from build123d import *


with BuildPart() as part:
    # Эскиз1 → Повернуть1 (revolve)
    with BuildSketch(Plane.XY):
        with BuildLine():
            Line((13.062177826, 3.5), (32, 12.5))
            Line((32, 12.5), (42, 12.5))
            Line((42, 12.5), (60.937822174, 3.5))
            ThreePointArc((60.937822174, 3.5), (68.811733316, 6.761480784), (74, 0))
            Line((74, 0), (0, 0))
            ThreePointArc((0, 0), (5.188266684, 6.761480784), (13.062177826, 3.5))
        make_face()
    revolve(axis=Axis((0, 0, 0), (1, 0, 0)))

    # Эскиз4 → Вырез-Повернуть1 (revolve, cut)
    with BuildSketch(Plane(origin=(37, 0, 0), x_dir=(0, 0, -1), z_dir=(1, 0, 0))):
        Polygon((-7.5, 10), (7.5, 10), (7.5, 20), (15, 20), (15, 0), (-15, 0), (-15, 20), (-7.5, 20), align=None)
    revolve(axis=Axis((37, 0, 0), (0, 0, -1)), mode=Mode.SUBTRACT)


solid = part.part
Verification items for the finished model (mm, model axes). A direction names the side the tool comes from. Coordinates: 2 decimals unless noted, no trailing zeros. Order: outer loops, then holes, each group sorted by start corner. A loop starts at its lowest first (then second) coordinate and runs counter-clockwise, first axis right, second up.
Item 1: Depth check by flat-ended pin: pin 1 (3 mm diameter, centred on y = -2.5, z = -3.5, fed in from -X); pin 2 (1 mm diameter, centred on x = 8.5, z = 5.5, fed in from -Y); pin 3 (2 mm diameter, centred on x = 49.5, z = 3, fed in from -Y). Enter the tip coordinate at first touch or a pass-through.
Filled in:
pin 1: stops at x = 0.58
pin 2: stops at y = -4.69
pin 3: stops at y = -9.01
Item 2: Material ranges on L1, parallel to X at y = 0, z = 0.25; L2, parallel to Y at x = 31, z = 2.75; L3, parallel to X at y = 0, z = 3.25, recorded low to high.
Filled in:
L1: x = 0 to 27, 47 to 74
L2: y = -11.71 to -8, 8 to 11.71
L3: x = 0.8 to 27, 47 to 73.2
Item 3: Section check B-B, the plane y = 0. Enter the section's corners in (x, z).
Filled in:
outline: (13.06, -3.5) - (21.48, -7.5) - (27, -7.5) - (27, 7.5) - (21.48, 7.5) - (13.06, 3.5) arc R7 ccw (long way) to start; (47, -7.5) - (52.52, -7.5) - (60.94, -3.5) arc R7 ccw (long way) to (60.94, 3.5) - (52.52, 7.5) - (47, 7.5) - close
Item 4: Release check for a two-part mould opening along X. For faces 1 (the face through (26, 0, 7.5)), 2 (the face through (18.455, -4.811, -3.689)) record: +X half, -X half, draft (parallel to the pull), parting line (faces both ways), or undercut.
Filled in:
face 1: draft
face 2: undercut
Item 5: Section check D-D, the plane z = -5. Give the number of separate pieces and of enclosed holes in the cut face, then the cut area to 3 significant figures.
Filled in:
separate pieces: 3
enclosed holes: 1
area: 504 mm2
Item 6: Access from +Z, -Z, +X, -X, +Y, -Y to the whole of each face (thin tool, end or side, straight path). Record for faces 3 (the face through (55.81, -4.711, -3.613)), 4 (the face through (26, 0, -7.5)).
Filled in:
face 3: none
face 4: -Z, +X, -X, +Y, -Y
Item 7: Section check C-C, the plane x = 38.5. Enter the section's corners in (y, z).
Filled in:
outline: (-10, -7.5) - (-9.89, -7.5) - (-9.89, 7.5) - (-10, 7.5) arc R12.5 ccw to start; (9.89, -7.5) - (10, -7.5) arc R12.5 ccw to (10, 7.5) - (9.89, 7.5) - close
Item 8: Section check A-A, the plane z = 0. Enter the section's corners in (x, y), then the cut area to 3 significant figures.
Filled in:
outline: (13.06, -3.5) - (32, -12.5) - (42, -12.5) - (60.94, -3.5) arc R7 ccw (long way) to (60.94, 3.5) - (42, 12.5) - (32, 12.5) - (13.06, 3.5) arc R7 ccw (long way) to start; hole circle Ø20 at (37, 0)
area: 841 mm2
